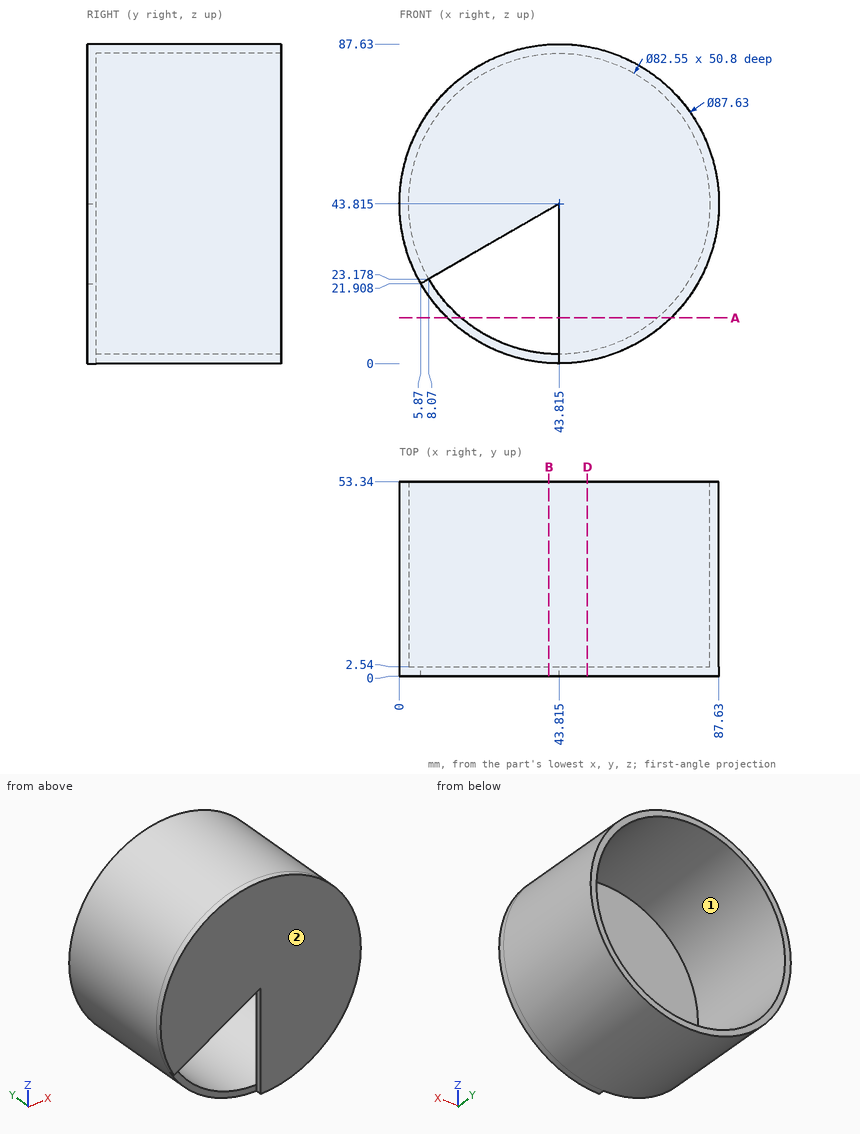
Here's the drawing with two shaded views (mm, measured from the low corner). I have some questions. Coordinates: 2 decimals unless noted, no trailing zeros. Loops run counter-clockwise (first coordinate to the right, second up) from the corner with the lowest first, then second, coordinate; pieces in that order, holes last. Notation, with made-up numbers: (40.5, 84) -> (51.5, 84) arc R19 ccw to (51.5, 99) -> close; hole circle Ø2 at (37.25, 50). An arc over 180 degrees is marked (long way). Answer as a JSON object with one key per item and string values.
1) Imagine slicing it at A-A (z = 12.5). Please give me the cut outline in (x, y) (1 decimal).
Results:
{"outline": "(13.2, 2.5) -> (16.9, 2.5) -> (16.9, 53.3) -> (13.2, 53.3) -> close; (43.8, 0) -> (74.5, 0) -> (74.5, 53.3) -> (70.7, 53.3) -> (70.7, 2.5) -> (43.8, 2.5) -> close"}
2) Thinking about a two-plate mould opening in X: for the marked faces 1 and 2, which applies, pulls with the +X half, pulls with the -X half, needs draft (parallel to the pull), parting line crosses it, or undercut?
Results:
{"face 1": "undercut", "face 2": "needs draft"}
3) Imagine slicing it at D-D (x = 51.5). Please give me the cut outline in (y, z).
Results:
{"outline": "(0, 0.68) -> (53.34, 0.68) -> (53.34, 3.26) -> (2.54, 3.26) -> (2.54, 84.37) -> (53.34, 84.37) -> (53.34, 86.95) -> (0, 86.95) -> close"}
4) Imagine slicing it at B-B (x = 41). Please give me the cut outline in (y, z).
Results:
{"outline": "(0, 42.19) -> (2.54, 42.19) -> (2.54, 84.99) -> (53.34, 84.99) -> (53.34, 87.54) -> (0, 87.54) -> close; (2.54, 0.09) -> (53.34, 0.09) -> (53.34, 2.64) -> (2.54, 2.64) -> close"}
5) For P1, Ø12, axis at x = 14, y = 31.5, coming from the -Z side; P2, Ø8, axis at x = 23.5, y = 43, coming from the +Z side; P3, Ø18.5, axis at x = 26, z = 9.5, coming from the -Y side, each with a flat end and sliding along its axis, tell me the tip position at first contact or that it passes through.
Results:
{"P1": "stops at z = 7.04", "P2": "stops at z = 84.48", "P3": "stops at y = 2.54"}
6) If I drill on line 1 (Y direction, x = 65.5, z = 71); line 2 (Z direction, x = 14, y = 24) (1 decimal); line 3 (X direction, y = 22, z = 33.5), over which ranges is the centre line in solid material (lowest first)?
Results:
{"line 1": "y = 0 to 2.54", "line 2": "z = 11.7 to 15.3, 72.4 to 75.9", "line 3": "x = 1.23 to 3.85, 83.78 to 86.4"}
